```python
from build123d import *

# Parameters (mm, degrees)
SKETCH_1_W          = 25.5
SKETCH_1_H          = 20
SKETCH_1_W_2        = 22.5
SKETCH_1_H_2        = 17
EXTRUDE_1_DEPTH     = 16
M3X0_5_1_AT_2_COUNT = 2
M3X0_5_1_AT_2_PITCH = 17.755280905
EXTRUDE_2_REACH     = 32.529
SKETCH_4_R          = 7.5
EXTRUDE_3_DEPTH     = 13.8
SKETCH_6_R          = 2
EXTRUDE_4_DEPTH     = 7.6
SKETCH_7_R          = 2.2
EXTRUDE_5_DEPTH     = 11.2
SKETCH_9_R          = 2.363999551
EXTRUDE_6_DEPTH     = 18.4
SKETCH_10_R         = 1
CUT_EXTRUDE_1_DEPTH = 64.009285059
SKETCH_11_R         = 1
CUT_EXTRUDE_2_DEPTH = 18.4


with BuildPart() as part:
    # 草图1 → 凸台-拉伸1 (new body)
    with BuildSketch(Plane(origin=(0, 0, 0), x_dir=(1, 0, 0), z_dir=(0, 1, 0))):
        Rectangle(SKETCH_1_W, SKETCH_1_H)
        Rectangle(SKETCH_1_W_2, SKETCH_1_H_2, mode=Mode.SUBTRACT)
    extrude(amount=EXTRUDE_1_DEPTH)

    # 草图3 → M3x0.5 螺纹孔1 (revolve, cut)
    with BuildSketch(Plane(origin=(7.75, 12.75, 10), x_dir=(0, -1, 0), z_dir=(1, 0, 0))):
        Polygon((0, 0), (0, 1.5), (1.25, 1.5), (1.25, 0.275), (1.525, 0), align=None)
    m3x0_5_1 = revolve(axis=Axis((7.75, 12.75, 16.35), (0, 0, -1)), mode=Mode.SUBTRACT)

    # M3x0.5 螺纹孔1 at 2: M3x0.5 螺纹孔1 ×2
    with Locations(*[Vector(-0.8448190755542286, -0.5350520811843448, 0) * (i * M3X0_5_1_AT_2_PITCH) for i in range(1, M3X0_5_1_AT_2_COUNT)]):
        add(m3x0_5_1, mode=Mode.SUBTRACT)

    # 草图4 → 凸台-拉伸2 (add, up to next)
    with BuildSketch(Plane(origin=(-11.25, 0, 0), x_dir=(0, 0, -1), z_dir=(1, 0, 0)), mode=Mode.PRIVATE) as extrude_2_sk1:
        with Locations(Location((0, 8, 0), (0, 0, 180))):
            Circle(SKETCH_4_R)
    extrude_2_tool1 = extrude(extrude_2_sk1.sketch, amount=EXTRUDE_2_REACH, mode=Mode.PRIVATE) - part.part
    add(extrude_2_tool1.solids().sort_by_distance((-11.25, 8, 0))[0])

    # 草图5 → 凸台-拉伸3 (add)
    with BuildSketch(Plane.ZY.offset(12.75)):
        with BuildLine():
            ThreePointArc((-5.931717466, 10.266545369), (-6.35, 8), (-5.931717466, 5.733454631))
            ThreePointArc((-5.931717466, 5.733454631), (-6.363961031, 1.636038969), (-2.266545369, 2.068282534))
            ThreePointArc((-2.266545369, 2.068282534), (0, 1.65), (2.266545369, 2.068282534))
            ThreePointArc((2.266545369, 2.068282534), (6.363961031, 1.636038969), (5.931717466, 5.733454631))
            ThreePointArc((5.931717466, 5.733454631), (6.35, 8), (5.931717466, 10.266545369))
            ThreePointArc((5.931717466, 10.266545369), (6.363961031, 14.363961031), (2.266545369, 13.931717466))
            ThreePointArc((2.266545369, 13.931717466), (0, 14.35), (-2.266545369, 13.931717466))
            ThreePointArc((-2.266545369, 13.931717466), (-6.363961031, 14.363961031), (-5.931717466, 10.266545369))
        make_face()
    extrude(amount=EXTRUDE_3_DEPTH)

    # 草图6 → 凸台-拉伸4 (add)
    with BuildSketch(Plane(origin=(12.75, 0, 0), x_dir=(0, 0, -1), z_dir=(1, 0, 0))):
        with Locations(Location((0, 8, 0), (0, 0, 180))):
            Circle(SKETCH_6_R)
    extrude(amount=EXTRUDE_4_DEPTH)

    # 草图7 → 凸台-拉伸5 (add)
    with BuildSketch(Plane.ZY.offset(26.55)):
        with Locations((0, 8)):
            Circle(SKETCH_7_R)
    extrude(amount=EXTRUDE_5_DEPTH)

    # 草图9 → 凸台-拉伸6 (add)
    with BuildSketch(Plane.XY):
        with Locations((-19.65, 8)):
            Circle(SKETCH_9_R)
    extrude(amount=-EXTRUDE_6_DEPTH)

    # 草图10 → 切除-拉伸1 (cut, through all)
    with BuildSketch(Plane.ZY.offset(37.75)):
        with Locations((0, 8)):
            Circle(SKETCH_10_R)
    extrude(amount=-CUT_EXTRUDE_1_DEPTH, mode=Mode.SUBTRACT)

    # 草图11 → 切除-拉伸2 (cut)
    with BuildSketch(Plane(origin=(0, 0, -18.4), x_dir=(-1, 0, 0), z_dir=(0, 0, -1))):
        with Locations((19.65, 8)):
            Circle(SKETCH_11_R)
    extrude(amount=-CUT_EXTRUDE_2_DEPTH, mode=Mode.SUBTRACT)


solid = part.part
```
The listing builds one solid part. Answer for the finished solid, in the listing's coordinates (mm). A direction names the side the tool comes from. Coordinates: 2 decimals unless noted, no trailing zeros. Write each loop counter-clockwise with the first axis right and the second up, starting at its lowest first coordinate (ties: lowest second). Pieces come first, ordered by that corner, then holes. Notation, with made-up numbers: (-28, -34) - (-12, -34) arc R27 ccw to (-12, 5) - close; hole circle Ø9 at (-25, 72.25). An arc over 180 degrees is marked (long way). Return JSON: item names as keys, results as strings. Group by question number.
Q1. Which of the six approach directions +Z, -Z, +X, -X, +Y, -Y give full straight-line access (tool end or side, diameter ignored) to faces 5 (the flat face through (0, 8, -8.5)), 6 (the cylindrical face through (-20.19, 8.84, -9.33)), 7 (the cylindrical face through (8.51, 13.74, 9.12)), 8 (the cylindrical face through (-19.553, 14.317, 6.41))?
Q2. The part is cut by section D-D on z = -13.5. Write down the section's boundary in (x, y), and give its area (3 significant figures).
Q3. The part is cut by section C-C on x = -24. Write down the section's boundary in (y, z).
Q4. For a pull along Z with two mould halves and no side action, classify faces 1 (the cylindrical face through (-32.072, 9.855, 1.183)), 2 (the flat face through (11.25, 8, 8)), 3 (the cylindrical face through (-24.08, 8.03, -6.35)), 4 (the cylindrical face through (-17.47, 7.09, -12.08)) as +Z half, -Z half, draft (parallel to the pull), parting line (faces both ways), or undercut.
Q5. The part is cut by section A-A on x = -7.25. Write down the section's boundary in (y, z) (3 decimals).
Q6. Flat-ended cylindrical pins translate along their axes: pin 1 Ø5 at (y, z) = (7.5, -5) entering from +X; pin 2 Ø4 at (x, z) = (-18, -11.5) entering from -Y; pin 3 Ø6 at (x, z) = (-22.5, -9.5) entering from +Y. Find the tip coordinate at first contact, or state that the pin passes through.
Q7. The part is cut by section B-B on y = 8. State how many separate pieces and enclosed holes the cut face has, and give its area (3 significant figures).
Q8. Find the intervals of material crossed by line 1 along X through (y, z) = (8, -11.5); line 2 along Z through (x, y) = (9.5, 3.75); line 3 along Y through (x, z) = (-7.25, 9.25), in increasing order. Write a range as [from, to].
Evaluation:
{
 "1": {"face 5": "+Y, -Y", "face 6": "-Z", "face 7": "+Z", "face 8": "-X"},
 "2": {"outline": "circle Ø4.73 at (-19.65, 8); hole circle Ø2 at (-19.65, 8)", "area": "14.4 mm2"},
 "3": {"outline": "(2.07, -2.27) arc R2.65 ccw (long way) to (5.73, -5.93) arc R6.35 ccw to (10.27, -5.93) arc R2.65 ccw (long way) to (13.93, -2.27) arc R6.35 ccw to (13.93, 2.27) arc R2.65 ccw (long way) to (10.27, 5.93) arc R6.35 ccw to (5.73, 5.93) arc R2.65 ccw (long way) to (2.07, 2.27) arc R6.35 ccw to start; hole circle Ø2 at (8, 0)"},
 "4": {"face 1": "parting line", "face 2": "undercut", "face 3": "-Z half", "face 4": "draft"},
 "5": {"outline": "(0, -10) - (16, -10) - (16, -8.5) - (0, -8.5) - close; (0, 8.5) - (2, 8.5) - (2, 9.725) - (1.725, 10) - (0, 10) - close; circle Ø15 at (8, 0); (4.5, 8.5) - (16, 8.5) - (16, 10) - (4.775, 10) - (4.5, 9.725) - close; hole circle Ø2 at (8, 0)"},
 "6": {"pin 1": "stops at x = 12.75", "pin 2": "stops at y = 5.64", "pin 3": "stops at y = 14.22"},
 "7": {"separate pieces": "3", "enclosed holes": "2", "area": "626 mm2"},
 "8": {"line 1": "x = [-22.01, -20.65], [-18.65, -17.29]", "line 2": "z = [-10, -8.5], [-6.18, 6.18], [8.5, 10]", "line 3": "y = [0, 2], [4.5, 16]"}
}
